Answer from the drawing. Dimensions are ordinates in mm from the lowest x, y and z of the part. Round coordinates to 2 decimals unless told otherwise and drop trailing zeros. Loops run counter-clockwise (first coordinate to the right, second up) from the corner with the lowest first, then second, coordinate; pieces in that order, holes last. Notation, with made-up numbers: M -2.5,15.25 L 6.5,15.25 A19 ccw 6.5,43.25 Z; hole C 35,64 d8. An arc over 180 degrees is marked long. Write each question's results on one line, items separated by ' | '.
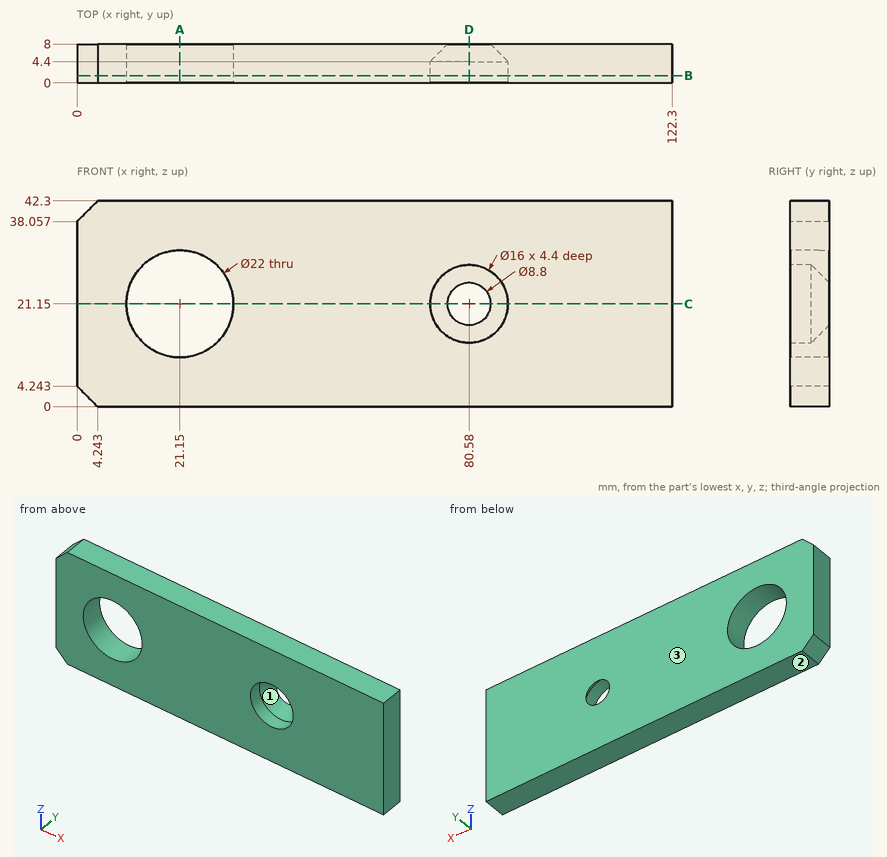
1. Find section C-C, the plane z = 21.15. Give the vertices of the cut face in (x, y).
Completed:
outline: M 0,0 L 10.15,0 L 10.15,8 L 0,8 Z; M 32.15,0 L 72.58,0 L 72.58,4.4 L 76.18,8 L 32.15,8 Z; M 84.98,8 L 88.58,4.4 L 88.58,0 L 122.3,0 L 122.3,8 Z
2. Find the intervals of material crossed by L1, parallel to X at y = 3, z = 21.15; L2, parallel to Z at x = 21.15, y = 6.5; L3, parallel to X at y = 0.75, z = 14.5 (1 decimal), in increasing order.
Completed:
L1: x = 0 to 10.15, 32.15 to 72.58, 88.58 to 122.3 | L2: z = 0 to 10.15, 32.15 to 42.3 | L3: x = 0 to 12.4, 29.9 to 76.1, 85 to 122.3
3. Find section B-B, the plane y = 1.5. Give the vertices of the cut face in (x, z), then the cut area to 3 significant figures.
Completed:
outline: M 0,4.24 L 4.24,0 L 122.3,0 L 122.3,42.3 L 4.24,42.3 L 0,38.06 Z; hole C 21.15,21.15 d22; hole C 80.58,21.15 d16 | area: 4,570 mm2
4. Find section D-D, the plane x = 80.58. Give the vertices of the cut face in (y, z), then the cut area to 3 significant figures.
Completed:
outline: M 0,0 L 8,0 L 8,16.75 L 4.4,13.15 L 0,13.15 Z; M 0,29.15 L 4.4,29.15 L 8,25.55 L 8,42.3 L 0,42.3 Z | area: 223 mm2
5. Given P1, Ø14.5, axis at x = 80.58, z = 21.15, coming from the -Y side, flat-ended and moving along its own axis, determine where the tip first touches the part or whether it passes through.
Completed:
P1: stops at y = 5.15
6. Determine the mould class of the marked faces 1, 2 and 3 for opening direction Z: released by +Z, released by -Z, zero draft, split by the parting line, or undercut.
Completed:
face 1: undercut | face 2: released by -Z | face 3: zero draft
7. Find section A-A, the plane x = 21.15. Give the vertices of the cut face in (y, z).
Completed:
outline: M 0,0 L 8,0 L 8,10.15 L 0,10.15 Z; M 0,32.15 L 8,32.15 L 8,42.3 L 0,42.3 Z
